Verification items for the finished model (mm, model axes). Give positions to 0.01 mm unless a question says otherwise; leave off trailing zeros. Write each loop counter-clockwise with the first axis right and the second up, starting at its lowest first coordinate (ties: lowest second). Pieces come first, ordered by that corner, then holes. Notation, with made-up numbers: M 15.5,18.25 L 64.5,18.25 A15 cw 64.5,37.25 Z; hole C 31.25,47.25 d8. An arc over 180 degrees is marked long. Write item = value, one per line.
from build123d import *

# Parameters (mm, degrees)
EXTRUDE_THIN1_DEPTH = 468.3125
FILLET1_R           = 1.27


with BuildPart() as part:
    # Sketch1 → Extrude-Thin1 (new body)
    with BuildSketch(Plane.XY):
        with BuildLine():
            Line((0, 46.83125), (-19.05, 46.83125))
            Line((-19.05, 46.83125), (-19.05, 30.1625))
            ThreePointArc((-19.05, 30.1625), (-10.631009886, 26.675240114), (-7.14375, 18.25625))
            Line((-7.14375, 18.25625), (-7.14375, 0))
            Line((-7.14375, 0), (0, 0))
            Line((0, 0), (0, 1.27))
            Line((0, 1.27), (-5.87375, 1.27))
            Line((-5.87375, 1.27), (-5.87375, 18.25625))
            ThreePointArc((-5.87375, 18.25625), (-9.294299063, 27.112878212), (-17.78, 31.371152366))
            Line((-17.78, 31.371152366), (-17.78, 45.56125))
            Line((-17.78, 45.56125), (0, 45.56125))
            Line((0, 45.56125), (0, 46.83125))
        make_face()
    extrude(amount=-EXTRUDE_THIN1_DEPTH)

    # Fillet1
    fillet1_edges = [part.edges().sort_by_distance(p)[0] for p in [
        (-7.14375, 0, -234.15625),
        (-19.05, 30.1625, -234.15625),
        (-19.05, 46.83125, -234.15625),
    ]]
    fillet(fillet1_edges, radius=FILLET1_R)


solid = part.part
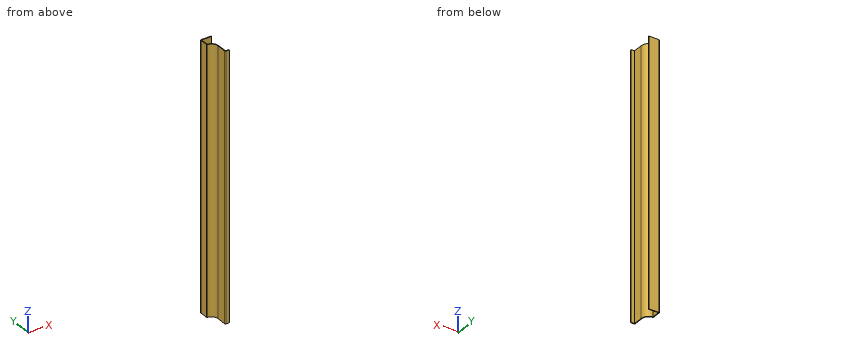
1) Material ranges on probe 1 along Y at (x, z) = (-2.5, -213.5); probe 2 along X at (y, z) = (34, -96.5); probe 3 along Y at (x, z) = (-12, -425), recorded low to high. Write a range as from..to.
From the geometry:
probe_1 = 0..1.27, 45.56..46.83
probe_2 = -19.05..-17.78
probe_3 = 27.85..29.39, 45.56..46.83
2) Depth check by flat-ended pin: P1, Ø18.5, axis at y = 9.5, z = -239, coming from the -X side; P2, Ø3, axis at y = 19.5, z = -130, coming from the +X side; P3, Ø10, axis at x = -14.5, y = 8, coming from the +Z side; P4, Ø15.5, axis at y = 36.5, z = -287.5, coming from the +X side. Enter the tip coordinate at first touch or a pass-through.
From the geometry:
P1 = -7.15
P2 = -5.87
P3 = through
P4 = -11.08
3) Cross-section at A-A on x = -11.5. Record the boundary of the cut face in (y, z), plus the area to 3 significant figures.
From the geometry:
outline = M 27.46,-468.31 L 29.05,-468.31 L 29.05,0 L 27.46,0 Z; M 45.56,-468.31 L 46.83,-468.31 L 46.83,0 L 45.56,0 Z
area = 1,340 mm^2
4) Cross-section at C-C on y = 10. Record the boundary of the cut face in (x, z).
From the geometry:
outline = M -7.14,-468.31 L -5.87,-468.31 L -5.87,0 L -7.14,0 Z
5) Cross-section at B-B on z = -317. Record the boundary of the cut face in (x, y).
From the geometry:
outline = M -19.05,31.37 A1.27 ccw -17.9,30.11 A11.91 cw -7.14,18.26 L -7.14,1.27 A1.27 ccw -5.87,0 L 0,0 L 0,1.27 L -5.87,1.27 L -5.87,18.26 A13.18 ccw -17.78,31.37 L -17.78,45.56 L 0,45.56 L 0,46.83 L -17.78,46.83 A1.27 ccw -19.05,45.56 Z
